Design review of the part built by this model. Coordinates are the model's own, in mm. A direction names the side the tool comes from. Give positions to 0.01 mm unless a question says otherwise; leave off trailing zeros. Write each loop counter-clockwise with the first axis right and the second up, starting at its lowest first coordinate (ties: lowest second). Pieces come first, ordered by that corner, then holes.
```python
from build123d import *

# Parameters (mm, degrees)
SKETCH1_W           = 42
SKETCH1_H           = 42
BOSS_EXTRUDE1_DEPTH = 19.5
CUT_EXTRUDE1_START  = -7.7
CUT_EXTRUDE1_DEPTH  = 22.9
SKETCH3_R           = 11
BOSS_EXTRUDE2_DEPTH = 2
CHAMFER1_SIZE       = 5
FILLET1_R           = 1
BOSS_EXTRUDE3_DEPTH = 16


with BuildPart() as part:
    # Sketch1 → Boss-Extrude1 (new, symmetric)
    with BuildSketch(Plane.XY):
        Rectangle(SKETCH1_W, SKETCH1_H)
    extrude(amount=BOSS_EXTRUDE1_DEPTH, both=True)

    # Sketch2 → Cut-Extrude1 (cut)
    with BuildSketch(Plane.XY.offset(19.5).offset(CUT_EXTRUDE1_START)):
        Polygon((-21, 21), (-13.5, 21), (-21, 13.5), align=None)
        Polygon((13.5, 21), (21, 21), (21, 13.5), align=None)
        Polygon((21, -13.5), (21, -21), (13.5, -21), align=None)
        Polygon((-13.5, -21), (-21, -21), (-21, -13.5), align=None)
    extrude(amount=-CUT_EXTRUDE1_DEPTH, mode=Mode.SUBTRACT)

    # Sketch3 → Boss-Extrude2 (add)
    with BuildSketch(Plane.XY.offset(19.5)):
        Circle(SKETCH3_R)
    extrude(amount=BOSS_EXTRUDE2_DEPTH)

    # Chamfer1
    chamfer1_edges = [part.edges().sort_by_distance(p)[0] for p in [
        (21, -21, -15.3),
        (-21, -21, -15.3),
        (-21, 21, -15.3),
        (21, 21, -15.3),
        (21, -21, 15.65),
        (-21, -21, 15.65),
        (-21, 21, 15.65),
        (21, 21, 15.65),
    ]]
    chamfer(chamfer1_edges, length=CHAMFER1_SIZE)

    # Fillet1
    fillet1_edges = [part.edges().sort_by_distance(p)[0] for p in [
        (-21, -13.5, 0.35),
        (-13.5, -21, 0.35),
        (13.5, -21, 0.35),
        (21, -13.5, 0.35),
        (21, 13.5, 0.35),
        (13.5, 21, 0.35),
        (-21, 13.5, 0.35),
        (-13.5, 21, 0.35),
        (-11, 0, 19.5),
        (0, 21, -19.5),
        (0, 21, 19.5),
        (-16, 21, 15.65),
        (-16, 21, -15.3),
        (16, 21, 15.65),
        (16, 21, -15.3),
        (21, 0, -19.5),
        (0, -21, -19.5),
        (-21, 0, -19.5),
        (-18.5, -18.5, -19.5),
        (-18.5, 18.5, -19.5),
        (18.5, -18.5, -19.5),
        (18.5, 18.5, -19.5),
        (21, 0, 19.5),
        (21, -16, -15.3),
        (21, -16, 15.65),
        (21, 16, 15.65),
        (21, 16, -15.3),
        (-21, 0, 19.5),
        (0, -21, 19.5),
        (-18.5, 18.5, 19.5),
        (-18.5, -18.5, 19.5),
        (18.5, -18.5, 19.5),
        (18.5, 18.5, 19.5),
        (-16, -21, 15.65),
        (-16, -21, -15.3),
        (16, -21, -15.3),
        (16, -21, 15.65),
        (-21, 16, 15.65),
        (-21, -16, 15.65),
        (-21, -16, -15.3),
        (-21, 16, -15.3),
    ]]
    fillet(fillet1_edges, radius=FILLET1_R)

    # Sketch4 → Boss-Extrude3 (add)
    with BuildSketch(Plane.XY.offset(21.5)):
        with BuildLine():
            Line((-2, -1.5), (-2, 1.5))
            ThreePointArc((-2, 1.5), (2.5, 0), (-2, -1.5))
        make_face()
    extrude(amount=BOSS_EXTRUDE3_DEPTH)


solid = part.part
```
(1) Clearance check with flat-ended pins moving along their axes: P1, Ø6.5, axis at x = 17.5, y = -16.5, coming from the +Z side; P2, Ø0.9, axis at y = 0, z = 30.5, coming from the -X side; P3, Ø12, axis at x = -15, y = 1, coming from the +Z side. State where each tip first meets the part, or that it passes through.
Resolved:
P1: stops at z = 19.5
P2: stops at x = -2
P3: stops at z = 21.5
(2) Consider section D-D, the plane z = -14. Give the boundary of the cut face in (x, y).
Resolved:
outline: (-21, -15.59) arc R1 ccw to (-20.71, -16.29) - (-16.29, -20.71) arc R1 ccw to (-15.59, -21) - (15.59, -21) arc R1 ccw to (16.29, -20.71) - (20.71, -16.29) arc R1 ccw to (21, -15.59) - (21, 15.59) arc R1 ccw to (20.71, 16.29) - (16.29, 20.71) arc R1 ccw to (15.59, 21) - (-15.59, 21) arc R1 ccw to (-16.29, 20.71) - (-20.71, 16.29) arc R1 ccw to (-21, 15.59) - close
(3) Tool access review of faces 1 (the face through (-18, 18, -11.1)), 2 (the face through (17.2, -17.3, 0.5)), 3 (the face through (-2, 0, 29)), 4 (the face through (9, -9, 19.5)): name each direction out of +Z, -Z, +X, -X, +Y, -Y from which nothing blocks a thin tool from reaching the whole face with its end or side.
Resolved:
face 1: -X, +Y
face 2: +X, -Y
face 3: +Z, -X, +Y, -Y
face 4: +Z
(4) Consider section A-A, the plane z = -7.5. Give the boundary of the cut face in (x, y).
Resolved:
outline: (-21, -13.09) arc R1 ccw to (-20.71, -13.79) - (-13.79, -20.71) arc R1 ccw to (-13.09, -21) - (13.09, -21) arc R1 ccw to (13.79, -20.71) - (20.71, -13.79) arc R1 ccw to (21, -13.09) - (21, 13.09) arc R1 ccw to (20.71, 13.79) - (13.79, 20.71) arc R1 ccw to (13.09, 21) - (-13.09, 21) arc R1 ccw to (-13.79, 20.71) - (-20.71, 13.79) arc R1 ccw to (-21, 13.09) - close
(5) To check wall thickness, follow L1, parallel to Z at x = 15, y = 15; L2, parallel to Z at x = -5, y = 9.5. State the ranges of each line that lie inside material, in increasing order.
Resolved:
L1: z = -19.5 to 19.5
L2: z = -19.5 to 21.5
(6) Consider section C-C, the plane y = 0. Give the boundary of the cut face in (x, z), then the cut area to 3 significant figures.
Resolved:
outline: (-21, -18.5) arc R1 ccw to (-20, -19.5) - (20, -19.5) arc R1 ccw to (21, -18.5) - (21, 18.5) arc R1 ccw to (20, 19.5) - (12, 19.5) arc R1 cw to (11, 20.5) - (11, 21.5) - (2.5, 21.5) - (2.5, 37.5) - (-2, 37.5) - (-2, 21.5) - (-11, 21.5) - (-11, 20.5) arc R1 cw to (-12, 19.5) - (-20, 19.5) arc R1 ccw to (-21, 18.5) - close
area: 1,750 mm2
(7) Consider section B-B, the plane x = 0. Give the boundary of the cut face in (y, z), then the cut area to 3 significant figures.
Resolved:
outline: (-21, -18.5) arc R1 ccw to (-20, -19.5) - (20, -19.5) arc R1 ccw to (21, -18.5) - (21, 18.5) arc R1 ccw to (20, 19.5) - (12, 19.5) arc R1 cw to (11, 20.5) - (11, 21.5) - (2.5, 21.5) - (2.5, 37.5) - (-2.5, 37.5) - (-2.5, 21.5) - (-11, 21.5) - (-11, 20.5) arc R1 cw to (-12, 19.5) - (-20, 19.5) arc R1 ccw to (-21, 18.5) - close
area: 1,760 mm2
